```python
from build123d import *

# Parameters (mm, degrees)
SKETCH2_R           = 3.429
BOSS_EXTRUDE1_DEPTH = 12.7


with BuildPart() as part:
    # Sketch2 → Boss-Extrude1 (new body)
    with BuildSketch(Plane.XY):
        with BuildLine():
            Line((-4.490128061, 22.450640303), (-10.840128061, 16.100640303))
            ThreePointArc((-10.840128061, 16.100640303), (-12.216635031, 14.040552038), (-12.7, 11.610512242))
            Line((-12.7, 11.610512242), (-12.7, -11.610512242))
            ThreePointArc((-12.7, -11.610512242), (-12.216635031, -14.040552038), (-10.840128061, -16.100640303))
            Line((-10.840128061, -16.100640303), (-4.490128061, -22.450640303))
            ThreePointArc((-4.490128061, -22.450640303), (0, -24.310512242), (4.490128061, -22.450640303))
            Line((4.490128061, -22.450640303), (22.450640303, -4.490128061))
            ThreePointArc((22.450640303, -4.490128061), (24.310512242, 0), (22.450640303, 4.490128061))
            Line((22.450640303, 4.490128061), (4.490128061, 22.450640303))
            ThreePointArc((4.490128061, 22.450640303), (0, 24.310512242), (-4.490128061, 22.450640303))
        make_face()
        with Locations((0, 15.875)):
            Circle(SKETCH2_R, mode=Mode.SUBTRACT)
        with Locations((15.875, 0)):
            Circle(SKETCH2_R, mode=Mode.SUBTRACT)
        with Locations((0, -15.875)):
            Circle(SKETCH2_R, mode=Mode.SUBTRACT)
        Polygon((6.35, 3.666174209), (0, 7.332348419), (-6.35, 3.666174209), (-6.35, -3.666174209), (0, -7.332348419), (6.35, -3.666174209), align=None, mode=Mode.SUBTRACT)
    extrude(amount=BOSS_EXTRUDE1_DEPTH)


solid = part.part
```
The listing builds one solid part. Answer for the finished solid, in the listing's coordinates (mm). A direction names the side the tool comes from. Give positions to 0.01 mm unless a question says otherwise; leave off trailing zeros. Order: outer loops, then holes, each group sorted by start corner. A loop starts at its lowest first (then second) coordinate and runs counter-clockwise, first axis right, second up. Notation, with made-up numbers: (13, 70) -> (18, 70) arc R6 cw to (18, 75) -> close; hole circle Ø10 at (33.25, -37). An arc over 180 degrees is marked (long way). Answer as a JSON object with one key per item and string values. Group by question number.
Item 1: The part is cut by section C-C on y = -13. Write down the section's boundary in (x, z).
Item 2: Consider L1, parallel to Y at x = 0, z = 2.5; L2, parallel to Y at x = -1, z = 2 (3 decimals); L3, parallel to X at y = 0.5, z = 5. Determine where each line is inside the solid, lowest interval first. Write a range as from..to.
Item 3: The part is cut by section A-A on x = 17.5. Write down the section's boundary in (y, z).
Item 4: The part is cut by section D-D on z = 10. Write down the section's boundary in (x, y) (3 decimals).
Item 5: Determine the mould class of faces 3 (the flat face through (13.6, 13.34, 6.26)), 4 (the cylindrical face through (0.07, 24.31, 6.26)), 5 (the flat face through (-3.131, 5.525, 6.261)) for opening direction X: pulls with the +X half, pulls with the -X half, needs draft (parallel to the pull), parting line crosses it, or undercut.
Item 6: The part is cut by section B-B on y = 0. Write down the section's boundary in (x, z).
Item 7: A tool of negligible diameter and unlimited length cuts with its end or side. For faces 1 (the flat face through (-6.35, 0, 6)), 2 (the flat face through (13.34, -13.6, 6.26)), from which of +Z, -Z, +X, -X, +Y, -Y can it reach the whole face along a straight path? Write none if from no direction.
Item 8: Flat-ended cylindrical pins translate along their axes: pin 1 (1 mm diameter, centred on y = 16, z = 2, fed in from -X); pin 2 (3 mm diameter, centred on y = -15.5, z = 7.5, fed in from -X). Find the tip coordinate at first contact, or state that the pin passes through.
Result set:
{
 "1": {"outline": "(-12.55, 0) -> (-1.87, 0) -> (-1.87, 12.7) -> (-12.55, 12.7) -> close; (1.87, 0) -> (13.94, 0) -> (13.94, 12.7) -> (1.87, 12.7) -> close"},
 "2": {"L1": "-24.31..-19.3, -12.45..-7.33, 7.33..12.45, 19.3..24.31", "L2": "-24.231..-19.155, -12.595..-6.755, 6.755..12.595, 19.155..24.231", "L3": "-12.7..-6.35, 6.35..12.48, 19.27..24.29"},
 "3": {"outline": "(-9.44, 0) -> (-3.02, 0) -> (-3.02, 12.7) -> (-9.44, 12.7) -> close; (3.02, 0) -> (9.44, 0) -> (9.44, 12.7) -> (3.02, 12.7) -> close"},
 "4": {"outline": "(-12.7, -11.611) arc R6.35 ccw to (-10.84, -16.101) -> (-4.49, -22.451) arc R6.35 ccw to (4.49, -22.451) -> (22.451, -4.49) arc R6.35 ccw to (22.451, 4.49) -> (4.49, 22.451) arc R6.35 ccw to (-4.49, 22.451) -> (-10.84, 16.101) arc R6.35 ccw to (-12.7, 11.611) -> close; hole (-6.35, -3.666) -> (0, -7.332) -> (6.35, -3.666) -> (6.35, 3.666) -> (0, 7.332) -> (-6.35, 3.666) -> close; hole circle Ø6.858 at (0, -15.875); hole circle Ø6.858 at (0, 15.875); hole circle Ø6.858 at (15.875, 0)"},
 "5": {"face 3": "pulls with the +X half", "face 4": "parting line crosses it", "face 5": "undercut"},
 "6": {"outline": "(-12.7, 0) -> (-6.35, 0) -> (-6.35, 12.7) -> (-12.7, 12.7) -> close; (6.35, 0) -> (12.45, 0) -> (12.45, 12.7) -> (6.35, 12.7) -> close; (19.3, 0) -> (24.31, 0) -> (24.31, 12.7) -> (19.3, 12.7) -> close"},
 "7": {"face 1": "+Z, -Z", "face 2": "+Z, -Z, +X, -Y"},
 "8": {"pin 1": "x = -11.37", "pin 2": "x = -12.23"}
}
